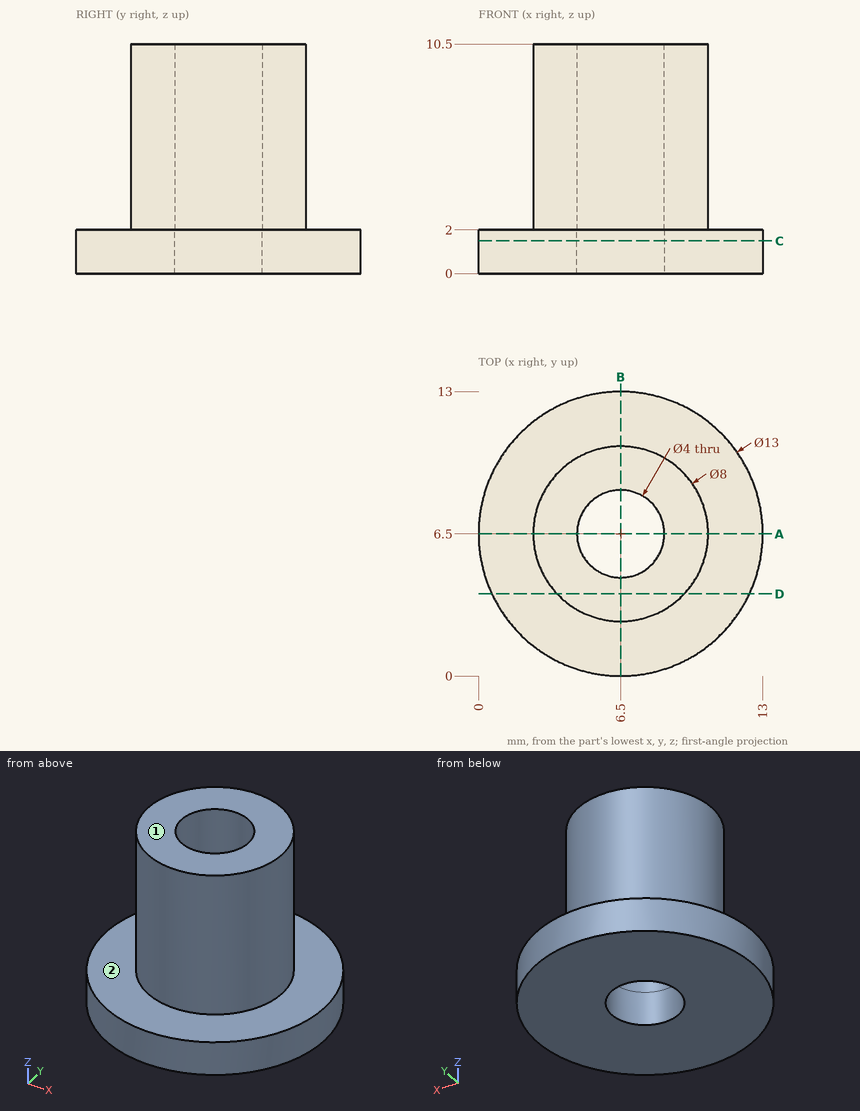
Design review of the part shown in the three views and the two pictorial views. Dimensions are in mm from the part's minimum x, y and z. A direction names the side the tool comes from. Give positions to 0.01 mm unless a question says otherwise; leave off trailing zeros. Write each loop counter-clockwise with the first axis right and the second up, starting at its lowest first coordinate (ties: lowest second). Pieces come first, ordered by that corner, then holes. Notation, with made-up numbers: (29.25, -40) - (79.25, -40) arc R15 cw to (79.25, -23) - close; hole circle Ø2 at (-38.5, 87.25). An arc over 180 degrees is marked (long way). Return JSON: item names as keys, results as strings. Group by question number.
(1) Machinability: for the marked faces 1 and 2, which of the approach directions +Z, -Z, +X, -X, +Y, -Y give a long, thin tool a straight path to every point of the face, cutting with its end or side? Answer none if there is none.
(2) To check wall thickness, follow probe 1 along Y at (x, z) = (6.5, 7); probe 2 along Y at (x, z) = (6.5, 1.25); probe 3 along Z at (x, y) = (1, 6). State the ranges of each line that lie inside material, in increasing order.
(3) We need section D-D, the plane y = 3.75. Give the boundary of the cut face in (x, z).
(4) We need section C-C, the plane z = 1.5. Give the boundary of the cut face in (x, y), then the cut area to 3 significant figures.
(5) We need section A-A, the plane y = 6.5. Give the boundary of the cut face in (x, z), then the cut area to 3 significant figures.
(6) Insertion check: pin 1 (1.5 mm diameter, centred on x = 3, y = 10.5, fed in from +Z); pin 2 (4 mm diameter, centred on x = 8, z = 5, fed in from -Y); pin 3 (3 mm diameter, centred on y = 4, z = 2.5, fed in from -X). Each pin has a flat end and moves straight along its axis. Give the tip position at first contact, or say it passes through.
Reported:
{
 "1": {"face 1": "+Z, +X, -X, +Y, -Y", "face 2": "+Z"},
 "2": {"probe 1": "y = 2.5 to 4.5, 8.5 to 10.5", "probe 2": "y = 0 to 4.5, 8.5 to 13", "probe 3": "z = 0 to 2"},
 "3": {"outline": "(0.61, 0) - (12.39, 0) - (12.39, 2) - (9.4, 2) - (9.4, 10.5) - (3.6, 10.5) - (3.6, 2) - (0.61, 2) - close"},
 "4": {"outline": "circle Ø13 at (6.5, 6.5); hole circle Ø4 at (6.5, 6.5)", "area": "120 mm2"},
 "5": {"outline": "(0, 0) - (4.5, 0) - (4.5, 10.5) - (2.5, 10.5) - (2.5, 2) - (0, 2) - close; (8.5, 0) - (13, 0) - (13, 2) - (10.5, 2) - (10.5, 10.5) - (8.5, 10.5) - close", "area": "52.0 mm2"},
 "6": {"pin 1": "stops at z = 2", "pin 2": "stops at y = 2.5", "pin 3": "stops at x = 0.09"}
}
